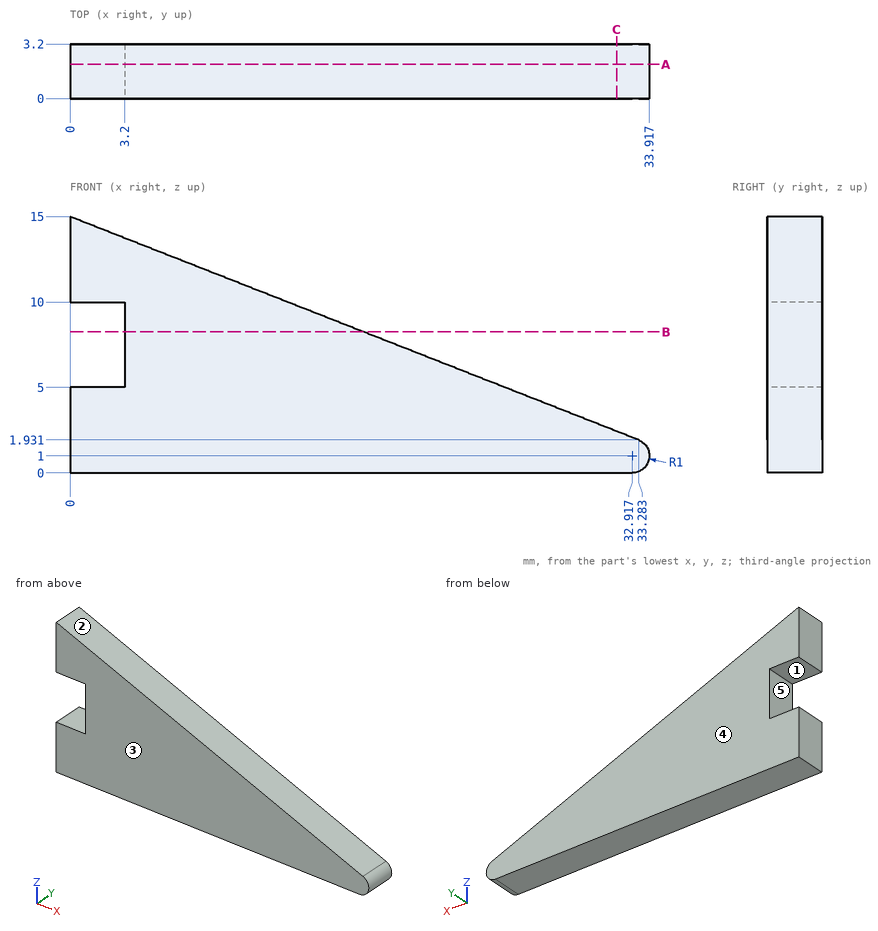
Here's the drawing with two shaded views (mm, measured from the low corner). I have some questions. A direction names the side the tool comes from. Give positions to 0.01 mm unless a question says otherwise; leave off trailing zeros. Order: outer loops, then holes, each group sorted by start corner. A loop starts at its lowest first (then second) coordinate and runs counter-clockwise, first axis right, second up.
Q1. If I drill on line 1 along Z through (x, y) = (2, 1.25) (1 decimal); line 2 along Z through (x, y) = (6.5, 2); line 3 along Z through (x, y) = (9.5, 1.75), over which ranges is the centre line in solid material (lowest first)?
Q2. For the marked faces 4 and 5, which set-ups out of +Z, -Z, +X, -X, +Y, -Y let a thin tool reach every point of the face, with its end or its side?
Q3. Suppose I cut it at B-B, the plane z = 8.25. Write out the boundary of the cut face in (x, y).
Q4. Suppose I cut it at A-A, the plane y = 2. Write out the boundary of the cut face in (x, z), and give its area (3 significant figures).
Q5. I'm going to push flat-ended pins straight in: P1, Ø8, axis at x = 17, z = 12, coming from the -Y side; P2, Ø1, axis at y = 1.5, z = 6.5, coming from the -X side; P3, Ø1.5, axis at x = 20, y = 2.5, coming from the +Z side. Where does each tip first touch, or does it pass through?
Q6. Suppose I cut it at C-C, the plane x = 32. Write out the boundary of the cut face in (y, z) (1 decimal).
Q7. We'd pull the mould along Z, two halves only. Please class the marked faces 1, 2 and 3: +Z half, -Z half, draft (parallel to the pull), parting line (faces both ways), or undercut.
Solution:
1. line 1: z = 0 to 5, 10 to 14.2
1. line 2: z = 0 to 12.45
1. line 3: z = 0 to 11.27
2. face 4: +Z, -Z, +X, -X, +Y
2. face 5: -X, +Y, -Y
3. outline: (3.2, 0) - (17.19, 0) - (17.19, 3.2) - (3.2, 3.2) - close
4. outline: (0, 0) - (32.92, 0) arc R1 ccw to (33.28, 1.93) - (0, 15) - (0, 10) - (3.2, 10) - (3.2, 5) - (0, 5) - close
4. area: 267 mm2
5. P1: stops at y = 0
5. P2: stops at x = 3.2
5. P3: stops at z = 7.44
6. outline: (0, 0) - (3.2, 0) - (3.2, 2.4) - (0, 2.4) - close
7. face 1: undercut
7. face 2: +Z half
7. face 3: draft
